Job drawing, mm, ordinate dimensions from the low corner. One solid piece. A direction names the side the tool comes from. Give positions to 0.01 mm unless a question says otherwise; leave off trailing zeros. Order: outer loops, then holes, each group sorted by start corner. A loop starts at its lowest first (then second) coordinate and runs counter-clockwise, first axis right, second up. Notation, with made-up numbers: M 49,4 L 72,4 A36 cw 72,38 Z; hole C 49.5,31 d9. An arc over 180 degrees is marked long. Put each result on its own line as item: value. Start each with the question number.
1) Cut at D-D (z = 19). Write the cut outline in (x, y), and give its area (3 significant figures).
2) Pin check, flat tips, straight feed: pin 1 (1.6 mm diameter, centred on x = 14, z = 1, fed in from -Y); pin 2 (13.5 mm diameter, centred on x = 50, y = 43, fed in from +Z); pin 3 (6 mm diameter, centred on x = 90, y = 43, fed in from -Z); pin 4 (3.5 mm diameter, centred on y = 1.5, z = 11, fed in from -X). Stop position of each tip, or through.
3) Cut at C-C (x = 60). Write the cut outline in (y, z), and give its area (3 significant figures).
4) Tool access for the marked faces 1 and 2: list every direction of +Z, -Z, +X, -X, +Y, -Y with a clear straight run to the whole face (end or side of a thin tool).
5) Drill centre lines: line 1 (Z direction, x = 90, y = 2.25); line 2 (Y direction, x = 130, z = 0.85); line 3 (Z direction, x = 48, y = 14). Where is each one in solid material? Low to high. Write a range as [from, to].
6) Cut at A-A (x = 10). Write the cut outline in (y, z).
7) Cut at B-B (z = 6). Write the cut outline in (x, y).
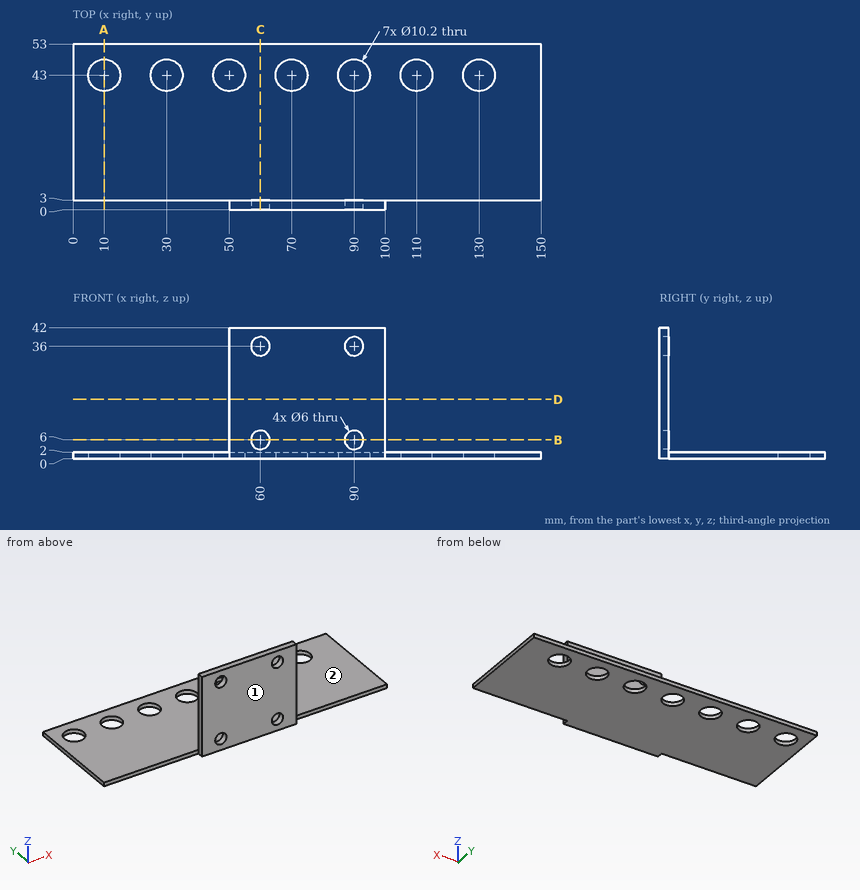
Solution:
1. outline: M 50,0 L 100,0 L 100,3 L 50,3 Z
1. area: 150 mm²
2. pin 1: y = 3
2. pin 2: z = 2
2. pin 3: through
2. pin 4: x = 50
3. outline: M 0,0 L 53,0 L 53,2 L 3,2 L 3,3 L 0,3 Z; M 0,9 L 3,9 L 3,33 L 0,33 Z; M 0,39 L 3,39 L 3,42 L 0,42 Z
3. area: 190 mm²
4. face 1: +Z, -Z, +X, -X, -Y
4. face 2: +Z, +X, -X, +Y
5. line 1: [0, 3], [9, 33], [39, 42]
5. line 2: [3, 37.9], [48.1, 53]
5. line 3: [0, 2]
6. outline: M 3,0 L 37.9,0 L 37.9,2 L 3,2 Z; M 48.1,0 L 53,0 L 53,2 L 48.1,2 Z
7. outline: M 50,0 L 57,0 L 57,3 L 50,3 Z; M 63,0 L 87,0 L 87,3 L 63,3 Z; M 93,0 L 100,0 L 100,3 L 93,3 Z
